The figure shows three views and two pictorial views of one solid part (mm, origin at its lowest corner). Answer the questions. A direction names the side the tool comes from. Coordinates: 2 decimals unless noted, no trailing zeros. Loops run counter-clockwise (first coordinate to the right, second up) from the corner with the lowest first, then second, coordinate; pieces in that order, holes last. Notation, with made-up numbers: (-9.75, 42) - (21.25, 42) arc R28 ccw to (21.25, 71) - close; hole circle Ø4 at (40.25, -28). An arc over 180 degrees is marked (long way). Return JSON: item names as keys, results as strings. Group by question number.
1. Which of the six approach directions +Z, -Z, +X, -X, +Y, -Y give full straight-line access (tool end or side, diameter ignored) to the marked faces 4 and 5?
2. Find the intervals of material crossed by line 1 along X through (y, z) = (57.5, 3.5); line 2 along Y through (x, z) = (59, 3.25); line 3 along Z through (x, y) = (86, 35.5), in increasing order.
3. Section C-C (y = 30.5) is taken. Write down the section's boundary in (x, z), and give its area (3 significant figures).
4. Section B-B (x = 14.5) is taken. Write down the section's boundary in (y, z), and give its area (3 significant figures).
5. This flat-tipped pin is pushed along its axis until it touches: P1, Ø1, axis at x = 47, y = 91, coming from the +Z side. Where does it stop, or does it pass through?
6. The mould has two halves that part along Y. Classify the marked faces 1, 2 and 3: pulls with the +Y half, pulls with the -Y half, needs draft (parallel to the pull), parting line crosses it, or undercut.
7. Section A-A (z = 13) is taken. Write down the section's boundary in (x, y).
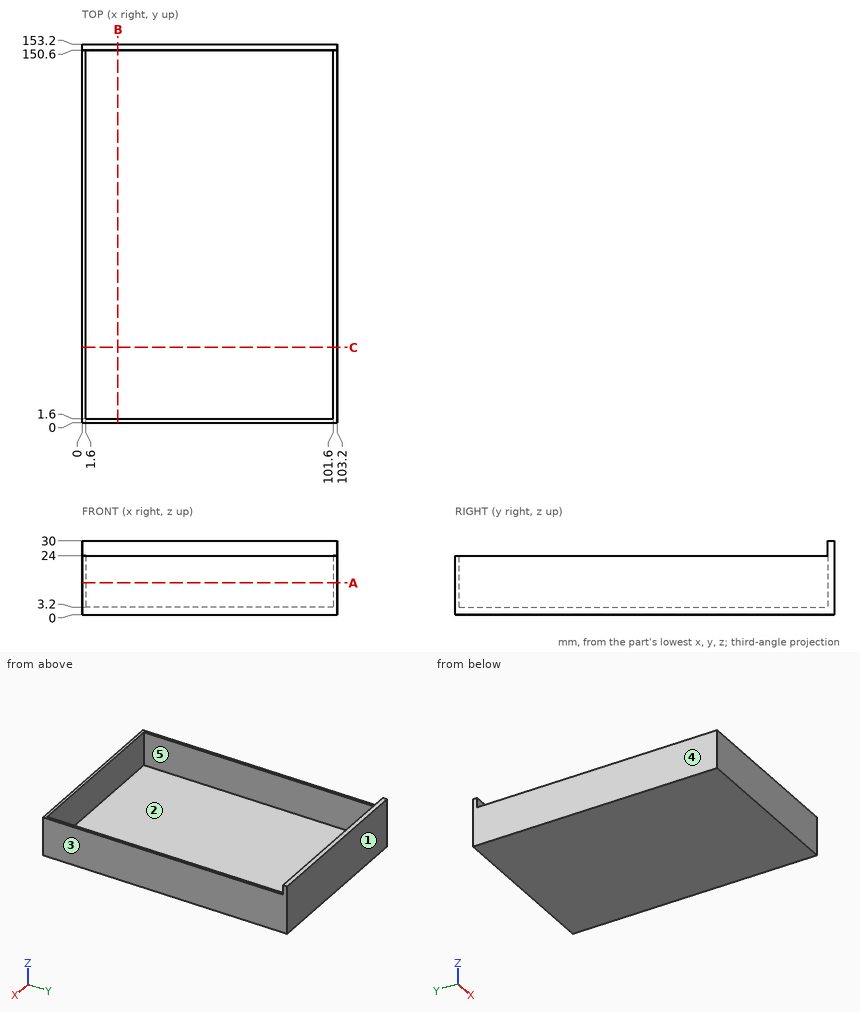
The answers:
{
 "1": {"face 4": "+Z, -Z, -X, +Y, -Y", "face 5": "+Z"},
 "2": {"line 1": "x = 0 to 1.6, 101.6 to 103.2", "line 2": "y = 0 to 1.6, 150.6 to 153.2", "line 3": "z = 0 to 3.2"},
 "3": {"outline": "(0, 0) - (103.2, 0) - (103.2, 24) - (101.6, 24) - (101.6, 3.2) - (1.6, 3.2) - (1.6, 24) - (0, 24) - close", "area": "397 mm2"},
 "4": {"outline": "(0, 0) - (153.2, 0) - (153.2, 30) - (150.6, 30) - (150.6, 3.2) - (1.6, 3.2) - (1.6, 24) - (0, 24) - close", "area": "593 mm2"},
 "5": {"P1": "stops at z = 3.2"},
 "6": {"face 1": "pulls with the +Y half", "face 2": "undercut", "face 3": "needs draft"},
 "7": {"outline": "(0, 0) - (103.2, 0) - (103.2, 153.2) - (0, 153.2) - close; hole (1.6, 1.6) - (101.6, 1.6) - (101.6, 150.6) - (1.6, 150.6) - close"}
}
